```python
from build123d import *

# Parameters (mm, degrees)
BOSS_EXTRUDE1_DEPTH = 5
CUT_EXTRUDE1_START  = -10
CUT_EXTRUDE1_DEPTH  = 10
FILLET2_R           = 3
SKETCH6_R           = 1.25
CUT_EXTRUDE2_DEPTH  = 3
CUT_EXTRUDE3_START  = -3
SKETCH7_R           = 1.25
CUT_EXTRUDE3_DEPTH  = 3


with BuildPart() as part:
    # Sketch1 → Boss-Extrude1 (new body)
    with BuildSketch(Plane(origin=(0, 0, 0), x_dir=(1, 0, 0), z_dir=(0, 1, 0))):
        with BuildLine():
            Line((-30, 0), (30, 0))
            ThreePointArc((30, 0), (0, 30), (-30, 0))
        make_face()
    extrude(amount=BOSS_EXTRUDE1_DEPTH)

    # Sketch5 → Cut-Extrude1 (cut)
    with BuildSketch(Plane(origin=(0, 5, 0), x_dir=(1, 0, 0), z_dir=(0, 1, 0)).offset(CUT_EXTRUDE1_START)):
        with BuildLine():
            Line((-21.580398915, 0), (-21.580398915, 5))
            Line((-21.580398915, 5), (-29.580398915, 5))
            ThreePointArc((-29.580398915, 5), (-29.894915684, 2.508787808), (-30, 0))
            Line((-30, 0), (-21.580398915, 0))
        make_face()
        with BuildLine():
            Line((21.580398915, 5), (29.580398915, 5))
            ThreePointArc((29.580398915, 5), (29.894915684, 2.508787808), (30, 0))
            Line((30, 0), (21.580398915, 0))
            Line((21.580398915, 0), (21.580398915, 5))
        make_face()
    extrude(amount=CUT_EXTRUDE1_DEPTH, mode=Mode.SUBTRACT)

    # Fillet2
    fillet2_edges = [part.edges().sort_by_distance(p)[0] for p in [
        (0, 5, 0),
    ]]
    fillet(fillet2_edges, radius=FILLET2_R)

    # Sketch6 → Cut-Extrude2 (cut)
    with BuildSketch(Plane(origin=(21.580398915, 0, 0), x_dir=(0, 0, -1), z_dir=(1, 0, 0))):
        with Locations((3, 2.25)):
            Circle(SKETCH6_R)
    extrude(amount=-CUT_EXTRUDE2_DEPTH, mode=Mode.SUBTRACT)

    # Sketch7 → Cut-Extrude3 (cut)
    with BuildSketch(Plane.ZY.offset(21.580398915).offset(CUT_EXTRUDE3_START)):
        with Locations(Location((-3, 2.25, 0), (0, 0, 180))):
            Circle(SKETCH7_R)
    extrude(amount=CUT_EXTRUDE3_DEPTH, mode=Mode.SUBTRACT)


solid = part.part
```
Source: CAD feature listing. Evaluate the final solid. Frame: model axes, mm. A direction names the side the tool comes from. Give positions to 0.01 mm unless a question says otherwise; leave off trailing zeros. Order: outer loops, then holes, each group sorted by start corner. A loop starts at its lowest first (then second) coordinate and runs counter-clockwise, first axis right, second up.
(1) Pull-direction query (Y, two-part tool) for faces 6 (the face through (-20.1, 1.9, -4.2)), 7 (the face through (0, 1, 0)), 8 (the face through (0.3, 4.1, -0.86)); classes: +Y half, -Y half, draft (parallel to the pull), parting line (faces both ways), or undercut.
(2) Access query for faces 1 (the face through (-21.58, 2, -1)), 2 (the face through (0, 5, -14)), 3 (the face through (21.58, 2, -1)), 4 (the face through (18.58, 2, -3)), 5 (the face through (-18.58, 2, -3)). Directions: +Z, -Z, +X, -X, +Y, -Y. A direction counts if a zero-diameter tool reaches every point of the face in a straight line with its end or side. Return the directions, or none.
(3) Section query C-C (z = -19.5). Return the cut outline in (x, y).
(4) Section query D-D (x = -24.5). Return the cut outline in (y, z), plus the area to 3 significant figures.
(5) Section query A-A (x = 3.5). Return the cut outline in (y, z), plus the area to 3 significant figures.
(6) Contact query for flat-ended pins moving along their axis: P1, Ø2, axis at y = 2.5, z = -3.5, coming from the -X side; P2, Ø1.5, axis at y = 1.5, z = -9, coming from the -X side; P3, Ø3, axis at y = 2.25, z = -3, coming from the +X side. Output: stop coordinate, or through.
(7) Section query B-B (y = 4.45). Return the cut outline in (x, z).
(8) Material intervals for line 1 along X through (y, z) = (2.55, -4.5); line 2 along Z through (x, y) = (-20.6, 2.25); line 3 along Z through (x, y) = (20, 3.15), sorted ascending.
Outcome:
1. face 6: undercut
1. face 7: draft
1. face 8: +Y half
2. face 1: +Z, -X, +Y, -Y
2. face 2: +Z, -Z, +X, -X, +Y
2. face 3: +Z, +X, +Y, -Y
2. face 4: +X
2. face 5: -X
3. outline: (-22.8, 0) - (22.8, 0) - (22.8, 5) - (-22.8, 5) - close
4. outline: (0, -17.31) - (5, -17.31) - (5, -5) - (0, -5) - close
4. area: 61.6 mm2
5. outline: (0, -29.8) - (5, -29.8) - (5, -3) arc R3 ccw to (2, 0) - (0, 0) - close
5. area: 147 mm2
6. P1: stops at x = -21.58
6. P2: stops at x = -28.84
6. P3: stops at x = 21.58
7. outline: (-29.58, -5) arc R30 ccw to (29.58, -5) - (21.58, -5) - (21.58, -1.27) - (-21.58, -1.27) - (-21.58, -5) - close
8. line 1: x = -21.58 to 21.58
8. line 2: z = -21.81 to -4.25, -1.75 to -0.01
8. line 3: z = -22.36 to -3.87, -2.13 to -0.23
